Source: three-view drawing plus pictorial views. Frame: mm from the lowest corner of the part. Round coordinates to 2 decimals unless told otherwise and drop trailing zeros. Loops run counter-clockwise (first coordinate to the right, second up) from the corner with the lowest first, then second, coordinate; pieces in that order, holes last. Notation, with made-up numbers: (-28, -19.5) -> (25, -19.5) arc R36 ccw to (25, 14.5) -> close; hole circle Ø5 at (59.5, 35.5). An arc over 180 degrees is marked (long way). Answer in a Markdown table with one row per item.
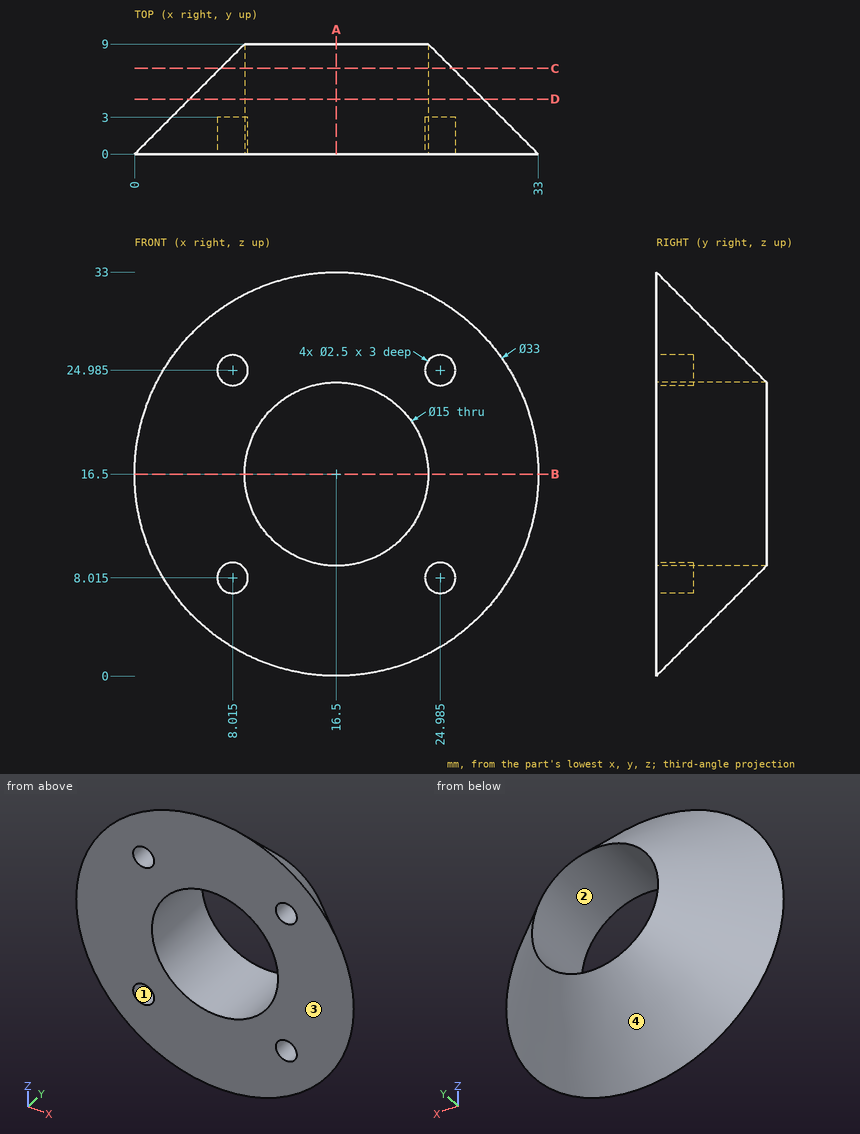
Item 1: Pin query (flat end, axial travel): pin 1 Ø1.5 at (x, z) = (29.5, 12.5) entering from +Y; pin 2 Ø3 at (y, z) = (7.5, 20) entering from +X (1 decimal); pin 3 Ø3 at (y, z) = (1.5, 27.5) entering from -X (1 decimal); pin 4 Ø9 at (x, z) = (16.5, 16.5) entering from +Y. Return the tip coordinate at first contact, or that it passes through.
Answer:
| item | result |
|---|---|
| pin 1 | stops at y = 3.65 |
| pin 2 | stops at x = 26.5 |
| pin 3 | stops at x = 3.8 |
| pin 4 | passes through |
Item 2: Cut plane C-C (y = 7). Output: boundary loops of the cut face in (x, z).
Answer:
| item | result |
|---|---|
| outline | circle Ø19 at (16.5, 16.5); hole circle Ø15 at (16.5, 16.5) |
Item 3: Cut plane B-B (z = 16.5). Output: boundary loops of the cut face in (x, y).
Answer:
| item | result |
|---|---|
| outline | (0, 0) -> (9, 0) -> (9, 9) -> close; (24, 0) -> (33, 0) -> (24, 9) -> close |
Item 4: Line query: probe 1 along X at (y, z) = (6, 21.5); probe 2 along X at (y, z) = (2.5, 16.5); probe 3 along Z at (x, y) = (15, 2.5). Output: solid intervals per line, ascending. Write a range as [from, to].
Answer:
| item | result |
|---|---|
| probe 1 | x = [7.27, 10.91], [22.09, 25.73] |
| probe 2 | x = [2.5, 9], [24, 30.5] |
| probe 3 | z = [2.58, 9.15], [23.85, 30.42] |
Item 5: Cut plane A-A (x = 16.5). Output: boundary loops of the cut face in (y, z), then the cut area to 3 significant figures.
Answer:
| item | result |
|---|---|
| outline | (0, 0) -> (9, 9) -> (0, 9) -> close; (0, 24) -> (9, 24) -> (0, 33) -> close |
| area | 81.0 mm² |
Item 6: Cut plane D-D (y = 4.5). Output: boundary loops of the cut face in (x, z).
Answer:
| item | result |
|---|---|
| outline | circle Ø24 at (16.5, 16.5); hole circle Ø15 at (16.5, 16.5) |
Item 7: Draft query along X for the marked faces 1, 2, 3 and 4. Return one class per face: pulls with the +X half, pulls with the -X half, needs draft (parallel to the pull), parting line crosses it, or undercut.
Answer:
| item | result |
|---|---|
| face 1 | undercut |
| face 2 | undercut |
| face 3 | needs draft |
| face 4 | parting line crosses it |
